Model file for the job. Use its own axes, mm. A direction names the side the tool comes from. Round coordinates to 2 decimals unless told otherwise and drop trailing zeros. Order: outer loops, then holes, each group sorted by start corner. A loop starts at its lowest first (then second) coordinate and runs counter-clockwise, first axis right, second up. Notation, with made-up numbers: (31.25, 43.25) - (66.25, 43.25) arc R18 cw to (66.25, 54.25) - close; hole circle Ø4 at (56.25, 56). An arc over 180 degrees is marked (long way). Answer as CSV lines item,"result". Start each with the question number.
1. Band-saw the part on C-C on y = -8.5. List the corners of the cut face in (x, z).
2. Band-saw the part on B-B on x = -33.5. List the corners of the cut face in (y, z).
3. Band-saw the part on A-A on z = 4.6. State how many separate pieces and enclosed holes the cut face has, then the cut area to 3 significant figures.
4. Pin check, flat tips, straight feed: pin 1 Ø2.5 at (x, z) = (-66, 3) entering from +Y; pin 2 Ø1.5 at (x, z) = (-25, 5) entering from -Y; pin 3 Ø1.2 at (y, z) = (-57, 2.5) entering from -X. Stop position of each tip, or through.
5. Wall check: line 1 along Y through (x, z) = (69, 2.65); line 2 along Y through (x, z) = (-4.09, 1.8); line 3 along X through (y, z) = (75, 2.75). Give the ranges that are in metal, low to high. Write a range as [from, to].
6. Pull direction X, two halves, no side cores. Call faces 1 (the face through (-60, -52, 3)), 2 (the face through (-22, -66, 3)), 3 (the face through (-3, 78, 3)): released by +X, released by -X, zero draft, split by the parting line, or undercut.
7. 3-axis set-ups, long thin cutter, end or side, ignore diameter. For faces 4 (the face through (-75, 38, 3)), 5 (the face through (-38, -69, 3)), 6 (the face through (-63, 56.2, 3)), 7 (the face through (-72, -63, 3)), 8 (the face through (69, 38, 3)): which of +Z, -Z, +X, -X, +Y, -Y reach the whole face in a straight line?
```python
from build123d import *

# Parameters (mm, degrees)
SKETCH1_R           = 1.75
BOSS_EXTRUDE2_DEPTH = 6


with BuildPart() as part:
    # Sketch1 → Boss-Extrude2 (new body)
    with BuildSketch(Plane.XY):
        Polygon((72, 72), (32, 72), (32, 78), (-38, 78), (-38, 72), (-72, 72), (-72, 56.2), (-67.772810154, 56.2), (-67.772810154, 57.6), (-64.957983727, 57.6), (-64.957983727, 56.2), (-60, 56.2), (-60, 53), (-64.957983727, 53), (-64.957983727, 51.568504207), (-67.772810154, 51.568504207), (-67.772810154, 53), (-72, 53), (-72, 38), (-78, 38), (-78, -32), (-72, -32), (-72, -50.4), (-67.78187279, -50.4), (-67.78187279, -49), (-64.967046362, -49), (-64.967046362, -50.4), (-60, -50.4), (-60, -53.6), (-64.967046362, -53.6), (-64.967046362, -55), (-67.78187279, -55), (-67.78187279, -53.6), (-72, -53.6), (-72, -72), (-38, -72), (-38, -66), (-4.6, -66), (-4.6, -61), (-6, -61), (-6, -58), (-4.6, -58), (-4.6, -54), (-1.4, -54), (-1.4, -58), (0, -58), (0, -61), (-1.4, -61), (-1.4, -66), (32, -66), (32, -72), (72, -72), (72, -32), (66, -32), (66, 38), (72, 38), align=None)
        with Locations((69, -52)):
            Circle(SKETCH1_R, mode=Mode.SUBTRACT)
        with Locations((69, 55)):
            Circle(SKETCH1_R, mode=Mode.SUBTRACT)
        with Locations((-4.09, 75)):
            Circle(SKETCH1_R, mode=Mode.SUBTRACT)
    extrude(amount=BOSS_EXTRUDE2_DEPTH)


solid = part.part
```
Reply:
1,outline,"(-78, 0) - (66, 0) - (66, 6) - (-78, 6) - close"
2,outline,"(-66, 0) - (78, 0) - (78, 6) - (-66, 6) - close"
3,separate pieces,"1"
3,enclosed holes,"3"
3,area,"20,600 mm2"
4,pin 1,"stops at y = 72"
4,pin 2,"stops at y = -66"
4,pin 3,"stops at x = -72"
5,line 1,"y = [-72, -53.75], [-50.25, -32], [38, 53.25], [56.75, 72]"
5,line 2,"y = [-54, 73.25], [76.75, 78]"
5,line 3,"x = [-38, -5.84], [-2.34, 32]"
6,face 1,"released by -X"
6,face 2,"undercut"
6,face 3,"zero draft"
7,face 4,"+Z, -Z, -X, +Y"
7,face 5,"+Z, -Z, -Y"
7,face 6,"+Z, -Z, -X"
7,face 7,"+Z, -Z, -X, -Y"
7,face 8,"+Z, -Z, +X"
